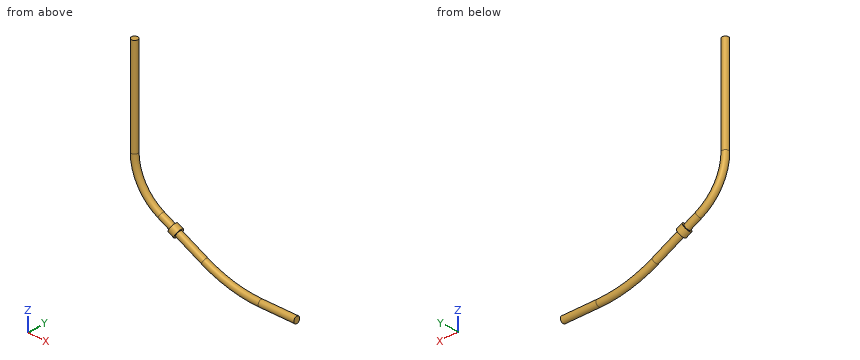
```python
from build123d import *

# Parameters (mm, degrees)
ESQUISSE2_R        = 1
ESQUISSE3_R        = 1.5
ESQUISSE3_R_2      = 1
EXTRU_MINCE1_DEPTH = 1


with BuildPart() as part:
    # Balayage1: sweep along a path in Esquisse1
    with BuildLine(Plane(origin=(0, 0, 0), x_dir=(1, 0, 0), z_dir=(0, 1, 0))) as balayage1_path:
        Line((0, 0), (0, 30))
        ThreePointArc((0, 30), (2.22403872, 37.8596955), (8.236641781, 43.388688719))
        Line((8.236641781, 43.388688719), (21.6253305, 50.152046937))
        ThreePointArc((21.6253305, 50.152046937), (30.076611959, 53.244881504), (39.014580281, 54.29488448))
        Line((39.014580281, 54.29488448), (50, 54.29488448))
    # Esquisse2 → Balayage1 (sweep)
    with BuildSketch(Plane.XY):
        Circle(ESQUISSE2_R)
    sweep(path=balayage1_path.line)

    # Esquisse3 → Extru.-Mince1 (add, symmetric)
    with BuildSketch(Plane(origin=(28.487028331, 0, -14.390354518), x_dir=(0.450890548, 0, 0.892579248), z_dir=(-0.892579248, 0, 0.450890548))):
        with Locations((-35.014019219, 0)):
            Circle(ESQUISSE3_R)
        with Locations((-35.014019219, 0)):
            Circle(ESQUISSE3_R_2, mode=Mode.SUBTRACT)
    extrude(amount=EXTRU_MINCE1_DEPTH, both=True)


solid = part.part
```
Source: CAD feature listing. Evaluate the final solid. Frame: model axes, mm. Round coordinates to 2 decimals unless told otherwise and drop trailing zeros. Loops run counter-clockwise (first coordinate to the right, second up) from the corner with the lowest first, then second, coordinate; pieces in that order, holes last.
1. Ray query, L1, parallel to X at y = -0.6, z = -29.5; L2, parallel to X at y = -0.2, z = -24.5; L3, parallel to Z at x = 38, y = -0.9. Return the intervals inside material, ascending.
2. Section query B-B on y = 0. Output: boundary loops of the cut face in (x, z).
3. Section query C-C on x = 42.5. Output: boundary loops of the cut face in (y, z).
4. Section query A-A on z = -28.5. Output: boundary loops of the cut face in (x, y), and give its area (3 significant figures).
Answers below:
1. L1: x = -0.8 to 0.8
1. L2: x = -0.98 to 0.98
1. L3: z = -54.72 to -53.85
2. outline: (-1, -30) arc R16 ccw to (7.79, -44.28) - (11.36, -46.08) - (11.13, -46.53) - (12.92, -47.43) - (13.14, -46.99) - (21.17, -51.04) arc R39.57 ccw to (39.01, -55.29) - (50, -55.29) - (50, -53.29) - (39.01, -53.29) arc R37.57 cw to (22.08, -49.26) - (14.04, -45.2) - (14.27, -44.76) - (12.48, -43.85) - (12.26, -44.3) - (8.69, -42.5) arc R14 cw to (1, -30) - (1, 0) - (-1, 0) - close
3. outline: circle Ø2 at (0, -54.29)
4. outline: circle Ø2 at (0, 0)
4. area: 3.14 mm2
